Design review of the part shown in the three views and the two pictorial views. Dimensions are in mm from the part's minimum x, y and z. Coordinates: 2 decimals unless noted, no trailing zeros. Write each loop counter-clockwise with the first axis right and the second up, starting at its lowest first coordinate (ties: lowest second). Pieces come first, ordered by that corner, then holes. Notation, with made-up numbers: (43.25, -24) - (51.25, -24) arc R22 ccw to (51.25, -7) - close; hole circle Ø5 at (22.5, 26.25). An arc over 180 degrees is marked (long way). Return JSON: item names as keys, results as strings. Group by question number.
(1) To check wall thickness, follow L1, parallel to Y at x = 44.45, z = 6; L2, parallel to X at y = 292.1, z = 6.25; L3, parallel to Y at x = 41, z = 2.25. State the ranges of each line that lie inside material, in increasing order. Write a range as from..to.
(2) We need section A-A on x = 44.45. State the section outline as (y, z) points, then the cut area to 3 significant figures.
(3) For pin 1 Ø7.5 at (x, y) = (44.45, 38.1) entering from -Z, flat-tipped, find the tip position at first contact; note if it passes through.
(4) We need section B-B on y = 292.1. State the section outline as (x, z) points, then the cut area to 3 significant figures.
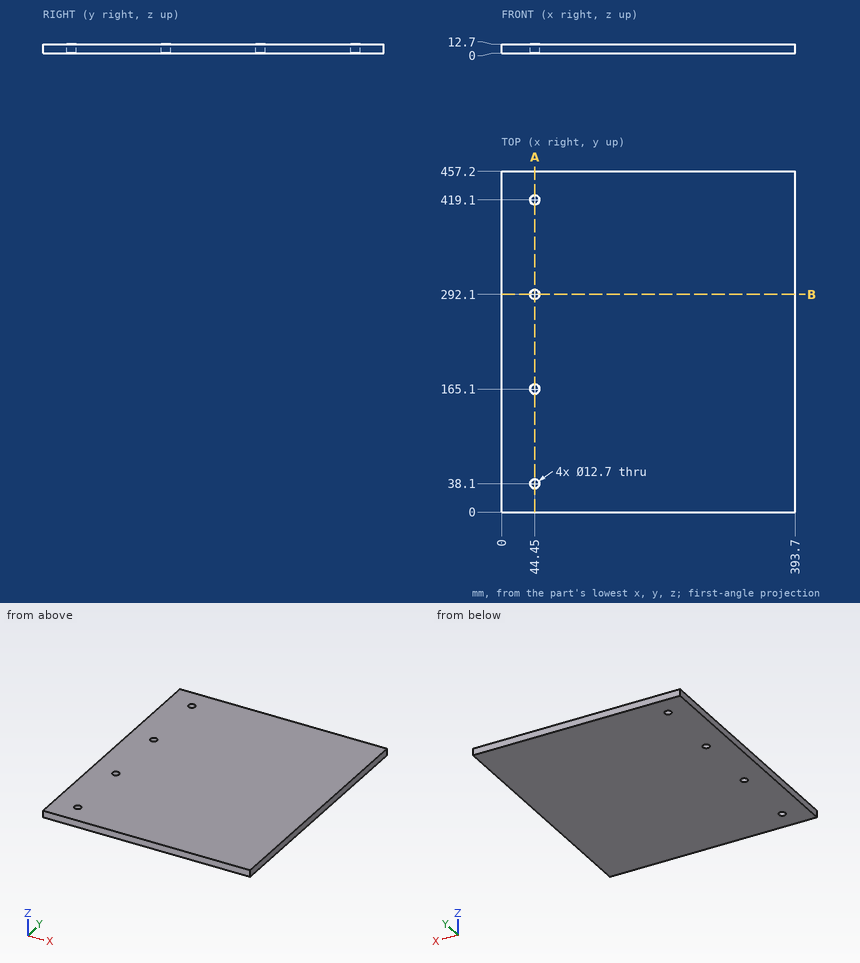
Ans:
{
 "1": {"L1": "0..31.75, 44.45..158.75, 171.45..285.75, 298.45..412.75, 425.45..457.2", "L2": "0..38.1, 50.8..393.7", "L3": "0..32.77, 43.43..159.77, 170.43..286.77, 297.43..413.77, 424.43..457.2"},
 "2": {"outline": "(0, 0) - (31.75, 0) - (31.75, 12.7) - (0, 12.7) - close; (44.45, 0) - (158.75, 0) - (158.75, 12.7) - (44.45, 12.7) - close; (171.45, 0) - (285.75, 0) - (285.75, 12.7) - (171.45, 12.7) - close; (298.45, 0) - (412.75, 0) - (412.75, 12.7) - (298.45, 12.7) - close; (425.45, 0) - (457.2, 0) - (457.2, 12.7) - (425.45, 12.7) - close", "area": "5,160 mm²"},
 "3": {"pin 1": "through"},
 "4": {"outline": "(0, 0) - (38.1, 0) - (38.1, 12.7) - (0, 12.7) - close; (50.8, 0) - (393.7, 0) - (393.7, 12.7) - (50.8, 12.7) - close", "area": "4,840 mm²"}
}
